from build123d import *

# Parameters (mm, degrees)
F1_DEPTH      = 20
F3_DEPTH      = 5
F3_DEPTH_BACK = 5


with BuildPart() as f1:
    # F0 (on Front) → F1 (new body)
    with BuildSketch(Plane.XZ):
        Polygon((-58.466492, 25), (-58.466492, 0), (-58.466492, -25), (41.533508, -25), (41.533508, 0), (33.533508, 8), (33.533508, 0), (24.533508, 0), (24.533508, 17), (16.533508, 25), (16.533508, 0), (8.533508, 8), (8.533508, 0), (-0.466492, 0), (-0.466492, 17), (-8.466492, 25), (-8.466492, 0), (-16.466492, 8), (-16.466492, 0), (-25.466492, 0), (-25.466492, 17), (-33.466492, 25), (-33.466492, 0), (-41.466492, 8), (-41.466492, 0), (-50.466492, 0), (-50.466492, 17), align=None)
        Polygon((33.533508, 0), (33.533508, 8), (24.533508, 17), (24.533508, 0), align=None)
        Polygon((8.533508, 0), (8.533508, 8), (-0.466492, 17), (-0.466492, 0), align=None)
        Polygon((-16.466492, 8), (-25.466492, 17), (-25.466492, 0), (-16.466492, 0), align=None)
        Polygon((-41.466492, 8), (-50.466492, 17), (-50.466492, 0), (-41.466492, 0), align=None)
    extrude(amount=F1_DEPTH)


with BuildPart() as f1_1:
    # F2: moved
    add(f1.part.moved(Location((0, 10, 0))))

    # F0 (on Front) → F3 (cut, two sides)
    with BuildSketch(Plane.XZ) as f3_sk:
        Polygon((33.533508, 0), (33.533508, 8), (24.533508, 17), (24.533508, 0), align=None)
        Polygon((8.533508, 0), (8.533508, 8), (-0.466492, 17), (-0.466492, 0), align=None)
        Polygon((-16.466492, 8), (-25.466492, 17), (-25.466492, 0), (-16.466492, 0), align=None)
        Polygon((-41.466492, 8), (-50.466492, 17), (-50.466492, 0), (-41.466492, 0), align=None)
    extrude(amount=F3_DEPTH, mode=Mode.SUBTRACT)
    extrude(f3_sk.sketch, amount=-F3_DEPTH_BACK, mode=Mode.SUBTRACT)


solid = f1_1.part
Read the model definition and answer for the solid it produces. Units are mm, in the model's axes. A direction names the side the tool comes from. Coordinates: 2 decimals unless noted, no trailing zeros. Write each loop counter-clockwise with the first axis right and the second up, starting at its lowest first coordinate (ties: lowest second). Pieces come first, ordered by that corner, then holes. Notation, with made-up numbers: (82.5, 67) -> (87.5, 67) arc R20 cw to (87.5, 73) -> close; hole circle Ø8 at (66, 57.5). An arc over 180 degrees is marked (long way). Return JSON: item names as keys, results as strings.
(1) The part is cut by section C-C on x = 29.5. Give the vertices of the cut face in (y, z).
Answers below:
{"outline": "(-10, -25) -> (10, -25) -> (10, 12.03) -> (5, 12.03) -> (5, 0) -> (-5, 0) -> (-5, 12.03) -> (-10, 12.03) -> close"}
(2) Which of the six approach directions +Z, -Z, +X, -X, +Y, -Y give full straight-line access (tool end or side, diameter ignored) to faces 1 (the flat face through (-8.466, 0, 13)), 2 (the flat face through (29.209, 6.807, 12.325)), 3 (the flat face through (28, 5, 7))?
Answers below:
{"face 1": "+Z, +Y, -Y", "face 2": "+Z, +X, +Y, -Y", "face 3": "+Z"}
(3) The part is cut by section A-A on z = 18. Give the vertices of the cut face in (x, y).
Answers below:
{"outline": "(-58.47, -10) -> (-51.47, -10) -> (-51.47, 10) -> (-58.47, 10) -> close; (-33.47, -10) -> (-26.47, -10) -> (-26.47, 10) -> (-33.47, 10) -> close; (-8.47, -10) -> (-1.47, -10) -> (-1.47, 10) -> (-8.47, 10) -> close; (16.53, -10) -> (23.53, -10) -> (23.53, 10) -> (16.53, 10) -> close"}
(4) For a pull along X with two mould halves and no side action, classify faces 4 (the flat face through (-58.466, 0, 0)), 5 (the flat face through (-22, -5, 7)), 6 (the flat face through (-9, 10, -5)) as pulls with the +X half, pulls with the -X half, needs draft (parallel to the pull), parting line crosses it, or undercut.
Answers below:
{"face 4": "pulls with the -X half", "face 5": "undercut", "face 6": "needs draft"}
(5) The part is cut by section D-D on y = 8. Give the vertices of the cut face in (x, z).
Answers below:
{"outline": "(-58.47, -25) -> (41.53, -25) -> (41.53, 0) -> (16.53, 25) -> (16.53, 0) -> (-8.47, 25) -> (-8.47, 0) -> (-33.47, 25) -> (-33.47, 0) -> (-58.47, 25) -> close"}
(6) Consider line 1 along X through (y, z) = (-7.5, 10); line 2 along X through (y, z) = (-7.5, 6); line 3 along Z through (x, y) = (33.5, -5.75). Determine where each line is inside the solid, lowest interval first. Write a range as from..to.
Answers below:
{"line 1": "-58.47..-43.47, -33.47..-18.47, -8.47..6.53, 16.53..31.53", "line 2": "-58.47..-39.47, -33.47..-14.47, -8.47..10.53, 16.53..35.53", "line 3": "-25..8.03"}
(7) Each of these flat-tipped pins is pushed along its axis until it touches: P1, Ø8, axis at y = 2, z = 4.5, coming from the +X side; P2, Ø5, axis at y = 7.5, z = 9, coming from the +X side; P3, Ø10, axis at x = 30.5, y = -1.5, coming from the +Z side. Where does it stop, or does it pass through?
Answers below:
{"P1": "x = 41.03", "P2": "x = 35.03", "P3": "z = 14.6"}
(8) The part is cut by section B-B on y = 4. Give the vertices of the cut face in (x, z).
Answers below:
{"outline": "(-58.47, -25) -> (41.53, -25) -> (41.53, 0) -> (33.53, 8) -> (33.53, 0) -> (24.53, 0) -> (24.53, 17) -> (16.53, 25) -> (16.53, 0) -> (8.53, 8) -> (8.53, 0) -> (-0.47, 0) -> (-0.47, 17) -> (-8.47, 25) -> (-8.47, 0) -> (-16.47, 8) -> (-16.47, 0) -> (-25.47, 0) -> (-25.47, 17) -> (-33.47, 25) -> (-33.47, 0) -> (-41.47, 8) -> (-41.47, 0) -> (-50.47, 0) -> (-50.47, 17) -> (-58.47, 25) -> close"}
